from build123d import *

# Parameters (mm, degrees)
IZIM1_W                     = 28
IZIM1_H                     = 25
IZIM1_R                     = 1.25
Y_KSEKLIK_EKSTR_ZYON1_DEPTH = 2.5


with BuildPart() as part:
    # Çizim1 → Yükseklik-Ekstrüzyon1 (new body)
    with BuildSketch(Plane.YZ):
        with Locations((0, 9.6)):
            Rectangle(IZIM1_W, IZIM1_H)
        with Locations(Location((-10.87, 0, 0), (0, 0, 270))):
            Circle(IZIM1_R, mode=Mode.SUBTRACT)
        with Locations(Location((10.87, 0, 0), (0, 0, 270))):
            Circle(IZIM1_R, mode=Mode.SUBTRACT)
    extrude(amount=Y_KSEKLIK_EKSTR_ZYON1_DEPTH)


solid = part.part
The listing builds one solid part. Answer for the finished solid, in the listing's coordinates (mm). Give positions to 0.01 mm unless a question says otherwise; leave off trailing zeros. Write each loop counter-clockwise with the first axis right and the second up, starting at its lowest first coordinate (ties: lowest second). Pieces come first, ordered by that corner, then holes.
1) For a pull along Y with two mould halves and no side action, classify faces 1 (the face through (1.23, -9.63, 0.16)), 2 (the face through (0, 0, 10)), 3 (the face through (1, 14, 9)), 4 (the face through (1, -14, 9)) as pulls with the +Y half, pulls with the -Y half, needs draft (parallel to the pull), parting line crosses it, or undercut.
2) Find the intervals of material crossed by L1, parallel to Y at x = 0.55, z = 0; L2, parallel to Y at x = 0.45, z = 0.75; L3, parallel to Z at x = 2, y = 12, in increasing order.
3) Given P1, Ø2, axis at y = 10.87, z = 0, coming from the -X side; P2, Ø6, axis at y = -5.5, z = 7, coming from the -X side, each flat-ended and moving along its own axis, determine where each tip first touches the part or whether it passes through.
4) Section B-B (z = 0) is taken. Write down the section's boundary in (x, y).
5) Section A-A (y = -10.87) is taken. Write down the section's boundary in (x, z), and give its area (4 significant figures).
Response:
1. face 1: undercut
1. face 2: needs draft
1. face 3: pulls with the +Y half
1. face 4: pulls with the -Y half
2. L1: y = -14 to -12.12, -9.62 to 9.62, 12.12 to 14
2. L2: y = -14 to -11.87, -9.87 to 9.87, 11.87 to 14
2. L3: z = -2.9 to -0.53, 0.53 to 22.1
3. P1: passes through
3. P2: stops at x = 0
4. outline: (0, -14) - (2.5, -14) - (2.5, -12.12) - (0, -12.12) - close; (0, -9.62) - (2.5, -9.62) - (2.5, 9.62) - (0, 9.62) - close; (0, 12.12) - (2.5, 12.12) - (2.5, 14) - (0, 14) - close
5. outline: (0, -2.9) - (2.5, -2.9) - (2.5, -1.25) - (0, -1.25) - close; (0, 1.25) - (2.5, 1.25) - (2.5, 22.1) - (0, 22.1) - close
5. area: 56.25 mm2
